```python
from build123d import *

# Parameters (mm, degrees)
F0_W      = 25.3
F0_H      = 20
F1_DEPTH  = 5
F2_R      = 2.5
F3_DEPTH  = 5
F4_W      = 45
F4_H      = 60
F5_DEPTH  = 40
F6_W      = 54
F6_H      = 34
F7_DEPTH  = 42
F9_DEPTH  = 60
F10_W     = 58
F10_H     = 25
F11_DEPTH = 3
F12_W     = 17
F12_H     = 58
F13_DEPTH = 3
F14_R     = 1
F15_R     = 1
F17_DEPTH = 55
F18_R     = 3.5
F19_DEPTH = 10
F20_R     = 2
F21_DEPTH = 25
F23_DEPTH = 55


with BuildPart() as f1:
    # F0 (on Top) → F1 (new body, symmetric)
    with BuildSketch(Plane.XY):
        Rectangle(F0_W, F0_H)
    extrude(amount=F1_DEPTH, both=True)

    # F2 (on face) → F3 (cut)
    with BuildSketch(Plane(origin=(0, 0, -5), x_dir=(1, 0, 0), z_dir=(0, 0, -1))):
        with Locations((7.65, 5)):
            Circle(F2_R)
        with Locations((7.65, -5)):
            Circle(F2_R)
        with Locations((-7.65, -5)):
            Circle(F2_R)
        with Locations((-7.65, 5)):
            Circle(F2_R)
    extrude(amount=-F3_DEPTH, mode=Mode.SUBTRACT)

    # F4 (on face) → F5 (join)
    with BuildSketch(Plane.XY.offset(5)):
        with Locations((-9.85, 0)):
            Rectangle(F4_W, F4_H)
    extrude(amount=F5_DEPTH)

    # F6 (on face) → F7 (cut)
    with BuildSketch(Plane(origin=(-32.35, 0, 0), x_dir=(0, -1, 0), z_dir=(-1, 0, 0))):
        with Locations((0, 25)):
            Rectangle(F6_W, F6_H)
    extrude(amount=-F7_DEPTH, mode=Mode.SUBTRACT)

    # F8 (on face) → F9 (cut)
    with BuildSketch(Plane.XZ.offset(30)):
        Polygon((-27.766407865, 42), (-32.35, 42), (-32.35, 5), (-14.35, 5), (-27.766407865, 17), align=None)
    extrude(amount=-F9_DEPTH, mode=Mode.SUBTRACT)

    # F10 (on face) → F11 (cut)
    with BuildSketch(Plane(origin=(-27.766407865, 0, 0), x_dir=(0, -1, 0), z_dir=(-1, 0, 0))):
        with Locations((0, 29.5)):
            Rectangle(F10_W, F10_H)
    extrude(amount=-F11_DEPTH, mode=Mode.SUBTRACT)

    # F12 (on face) → F13 (cut)
    with BuildSketch(Plane(origin=(-3.8932578028, 0, -4.3527945505), x_dir=(0.7453559925, 0, -0.6666666667), z_dir=(-0.6666666667, 0, -0.7453559925))):
        with Locations((-23.5291918257, 0)):
            Rectangle(F12_W, F12_H)
    extrude(amount=-F13_DEPTH, mode=Mode.SUBTRACT)

    # F14
    f14_edges = [f1.edges().sort_by_distance(p)[0] for p in [
        (12.65, -30, 25),
        (-9.85, -30, 45),
        (12.65, 0, 45),
        (12.65, 30, 25),
        (-9.85, 30, 45),
    ]]
    fillet(f14_edges, radius=F14_R)

    # F15
    f15_edges = [f1.edges().sort_by_distance(p)[0] for p in [
        (-32.35, 0, 42),
        (-32.35, 0, 45),
        (-1.35, -30, 5),
        (-1.35, 30, 5),
    ]]
    fillet(f15_edges, radius=F15_R)

    # F16 (on face) → F17 (join)
    with BuildSketch(Plane.XZ.offset(-27)):
        Polygon((-21.1683316536, 42), (-24.766407865, 42), (-24.766407865, 40.5), (-23.766407865, 40.5), align=None)
    extrude(amount=F17_DEPTH)

    # F18 (on face) → F19 (join)
    with BuildSketch(Plane.YZ.offset(12.65)):
        with Locations((0, 25)):
            Circle(F18_R)
    extrude(amount=-F19_DEPTH)

    # F20 (on face) → F21 (cut)
    with BuildSketch(Plane(origin=(2.65, 0, 0), x_dir=(0, -1, 0), z_dir=(-1, 0, 0))):
        with Locations((0, 25)):
            Circle(F20_R)
    extrude(amount=-F21_DEPTH, mode=Mode.SUBTRACT)

    # F22 (on face) → F23 (join)
    with BuildSketch(Plane(origin=(0, -27, 0), x_dir=(-1, 0, 0), z_dir=(0, 1, 0))):
        Polygon((13.2041019662, 8), (14.322135955, 9), (10.2041019662, 8), align=None)
    extrude(amount=F23_DEPTH)


solid = f1.part
```
Geometry: final body of the model. Coordinates: model frame, mm. A direction names the side the tool comes from. Coordinates: 2 decimals unless noted, no trailing zeros. Loops run counter-clockwise (first coordinate to the right, second up) from the corner with the lowest first, then second, coordinate; pieces in that order, holes last. Notation, with made-up numbers: (16.5, 57.25) -> (65.5, 57.25) arc R5 cw to (65.5, 66.25) -> close; hole circle Ø2 at (-9.5, 47). An arc over 180 degrees is marked (long way). Use a Markdown table: item, result. Add a question column.
(1) Access query for faces 1 (the flat face through (-12.292, -0.378, 8.507)), 2 (the flat face through (-8, -5, 0)), 3 (the flat face through (2.65, 2, 23)), 4 (the flat face through (-28, 0, 42)), 5 (the flat face through (-12.65, 0, 0)). Directions: +Z, -Z, +X, -X, +Y, -Y. A direction counts if a zero-diameter tool reaches every point of the face in a straight line with its end or side. Return the directions, or none.
(2) Pin query (flat end, axial travel): pin 1 Ø7.5 at (y, z) = (0.5, 25) entering from -X; pin 2 Ø10 at (x, z) = (-25.5, 6) entering from +Y; pin 3 Ø2.5 at (x, y) = (7.5, 4.5) entering from -Z; pin 4 Ø1.1 at (x, y) = (-24.5, 4.5) entering from -Z. Return the tip coordinate at first contact, or that it passes through.
(3) Mould query, pull axis Z, two halves, no side actions, for faces 6 (the cylindrical face through (8, 0, 23)), 7 (the flat face through (-8, 5, 0)), 8 (the flat face through (0, 0, 8)), 9 (the cylindrical face through (-10.148, -5.11, -2.535)). Classes: pulls with the +Z half, pulls with the -Z half, needs draft (parallel to the pull), parting line crosses it, or undercut.
(4) Section query B-B, the plane x = 7.65. Return loops of the section in (y, z), plus the area to 3 significant figures.
(5) Line query: line 1 along X through (y, z) = (-5, -1); line 2 along Z through (x, y) = (9, 0); line 3 along Y through (x, z) = (6.5, 14). Output: solid intervals per line, ascending.
(6) Section query D-D, the plane y = 8.5. Return loops of the section in (x, z), plus the area to 3 significant figures.
(7) Section query C-C, the plane x = -3. Return loops of the section in (y, z).
(8) Section query A-A, the plane y = 0. Return loops of the section in (x, z), plus the area to 3 significant figures.
Answer:
| question | item | result |
|---|---|---|
| 1 | face 1 | none |
| 1 | face 2 | -Z |
| 1 | face 3 | -X |
| 1 | face 4 | -Z, -X |
| 1 | face 5 | -Z, -X, +Y, -Y |
| 2 | pin 1 | stops at x = 2.65 |
| 2 | pin 2 | passes through |
| 2 | pin 3 | stops at z = 0 |
| 2 | pin 4 | stops at z = 40.5 |
| 3 | face 6 | undercut |
| 3 | face 7 | pulls with the -Z half |
| 3 | face 8 | undercut |
| 3 | face 9 | needs draft |
| 4 | outline | (-30, 6) arc R1 ccw to (-29, 5) -> (-10, 5) -> (-10, -5) -> (-7.5, -5) -> (-7.5, 0) -> (-2.5, 0) -> (-2.5, -5) -> (2.5, -5) -> (2.5, 0) -> (7.5, 0) -> (7.5, -5) -> (10, -5) -> (10, 5) -> (29, 5) arc R1 ccw to (30, 6) -> (30, 44) arc R1 ccw to (29, 45) -> (-29, 45) arc R1 ccw to (-30, 44) -> close; circle Ø7 at (0, 25); hole (-27, 8) -> (27, 8) -> (27, 42) -> (-27, 42) -> close; hole circle Ø4 at (0, 25) |
| 4 | area | 739 mm^2 |
| 5 | line 1 | x = -12.65 to -10.15, -5.15 to 5.15, 10.15 to 12.65 |
| 5 | line 2 | z = -5 to 8, 21.5 to 23, 27 to 28.5, 42 to 45 |
| 5 | line 3 | y = -30 to -27, 27 to 30 |
| 6 | outline | (-32.35, 43) arc R1 ccw to (-31.35, 42) -> (-24.77, 42) -> (-24.77, 40.5) -> (-23.77, 40.5) -> (-21.17, 42) -> (9.65, 42) -> (9.65, 8) -> (-10.2, 8) -> (-14.32, 9) -> (-13.1, 7.9) -> (-15.1, 5.67) -> (-14.35, 5) -> (-12.65, 5) -> (-12.65, -5) -> (12.65, -5) -> (12.65, 44) arc R1 ccw to (11.65, 45) -> (-31.35, 45) arc R1 ccw to (-32.35, 44) -> close |
| 6 | area | 575 mm^2 |
| 7 | outline | (-30, 6) arc R1 ccw to (-29, 5) -> (-10, 5) -> (-10, -5) -> (10, -5) -> (10, 5) -> (29, 5) arc R1 ccw to (30, 6) -> (30, 44) arc R1 ccw to (29, 45) -> (-29, 45) arc R1 ccw to (-30, 44) -> close; hole (-27, 8) -> (27, 8) -> (27, 42) -> (-27, 42) -> close |
| 8 | outline | (-32.35, 43) arc R1 ccw to (-31.35, 42) -> (-24.77, 42) -> (-24.77, 40.5) -> (-23.77, 40.5) -> (-21.17, 42) -> (9.65, 42) -> (9.65, 28.5) -> (2.65, 28.5) -> (2.65, 27) -> (12.65, 27) -> (12.65, 44) arc R1 ccw to (11.65, 45) -> (-31.35, 45) arc R1 ccw to (-32.35, 44) -> close; (-15.1, 5.67) -> (-14.35, 5) -> (-12.65, 5) -> (-12.65, -5) -> (12.65, -5) -> (12.65, 23) -> (2.65, 23) -> (2.65, 21.5) -> (9.65, 21.5) -> (9.65, 8) -> (-10.2, 8) -> (-14.32, 9) -> (-13.1, 7.9) -> close |
| 8 | area | 584 mm^2 |
